```python
from build123d import *

# Parameters (mm, degrees)
BOSS_EXTRUDE1_DEPTH     = 50
CUT_EXTRUDE2_DEPTH      = 603.59853966
CUT_EXTRUDE2_DEPTH_BACK = 603.59853966
SKETCH3_W               = 40
SKETCH3_H               = 40


with BuildPart() as part:
    # Sketch1 → Boss-Extrude1 (new body)
    with BuildSketch(Plane.XY):
        Polygon((0, 0), (25, 14.43375673), (25, -585.56624327), (0, -600), (-25, -585.56624327), (-25, 14.43375673), align=None)
    extrude(amount=BOSS_EXTRUDE1_DEPTH)

    # Sketch3 → Cut-Extrude2 (cut, two sides: drawn at the far end of the back side and taken through both)
    with BuildSketch(Plane(origin=(0, 0, 0), x_dir=(1, 0, 0), z_dir=(0, 1, 0)).offset(-CUT_EXTRUDE2_DEPTH_BACK)):
        with Locations((0, -25)):
            Rectangle(SKETCH3_W, SKETCH3_H)
    extrude(amount=CUT_EXTRUDE2_DEPTH + CUT_EXTRUDE2_DEPTH_BACK, mode=Mode.SUBTRACT)


solid = part.part
```
Work out the finished part from the listing and answer in its coordinate system (mm). A direction names the side the tool comes from. Round coordinates to 2 decimals unless told otherwise and drop trailing zeros. Write each loop counter-clockwise with the first axis right and the second up, starting at its lowest first coordinate (ties: lowest second). Pieces come first, ordered by that corner, then holes. Notation, with made-up numbers: (6, -7) - (64, -7) arc R25 cw to (64, 23) - close; hole circle Ø4 at (40, -36). An arc over 180 degrees is marked (long way). Return JSON: item names as keys, results as strings. Group by question number.
Q1. Find the intervals of material crossed by L1, parallel to Z at x = 18, y = -49; L2, parallel to X at y = -483, z = 11.5; L3, parallel to Y at x = 23, z = 16.5, in increasing order.
Q2. This flat-tipped pin is pushed along its axis until it touches: pin 1 Ø3 at (x, z) = (16, 45) entering from -Y. Where does it stop, or does it pass through?
Q3. The part is cut by section A-A on z = 32.5. Write down the section's boundary in (x, y).
Q4. For faces 1 (the flat face through (21.01, -587.87, 24.65)), 2 (the flat face through (20.66, 11.93, 24.65)), 3 (the flat face through (20, -293, 25)), determine the directions among +Z, -Z, +X, -X, +Y, -Y from which every point of the face is accessible in a straight line to the end or side of a thin tool.
Q5. The part is cut by section B-B on x = -12. Write down the section's boundary in (y, z), then the cut area to 3 significant figures.
Q6. The part is cut by section C-C on y = -421.5. Write down the section's boundary in (x, z).
Q7. The mould has two halves that part along Z. Classify faces 4 (the flat face through (-25, -290, 25)), 5 (the flat face through (0, -288, 0)), 6 (the flat face through (-20, -293, 25)): released by +Z, released by -Z, zero draft, split by the parting line, or undercut.
Solved:
{
 "1": {"L1": "0 to 5, 45 to 50", "L2": "-25 to -20, 20 to 25", "L3": "-586.72 to 13.28"},
 "2": {"pin 1": "y = -591.63"},
 "3": {"outline": "(-25, -585.57) - (-20, -588.45) - (-20, 11.55) - (-25, 14.43) - close; (20, -588.45) - (25, -585.57) - (25, 14.43) - (20, 11.55) - close"},
 "4": {"face 1": "+Z, -Z, +X, -Y", "face 2": "+Z, -Z, +Y", "face 3": "+Y, -Y"},
 "5": {"outline": "(-593.07, 0) - (6.93, 0) - (6.93, 5) - (-593.07, 5) - close; (-593.07, 45) - (6.93, 45) - (6.93, 50) - (-593.07, 50) - close", "area": "6,000 mm²"},
 "6": {"outline": "(-25, 0) - (25, 0) - (25, 50) - (-25, 50) - close; hole (-20, 5) - (20, 5) - (20, 45) - (-20, 45) - close"},
 "7": {"face 4": "zero draft", "face 5": "released by -Z", "face 6": "undercut"}
}
